Could you check a few things on this model? Use its own coordinates, in mm. Face numbers are marked on the shaded views. A direction names the side the tool comes from. Round coordinates to 2 decimals unless told otherwise and drop trailing zeros. Write each loop counter-clockwise with the first axis right and the second up, starting at its lowest first coordinate (ties: lowest second). Pieces come first, ordered by that corner, then holes. Notation, with made-up numbers: (-26, -8) -> (-7, -8) arc R18 ccw to (-7, 6) -> close; hole circle Ø8 at (52, 42.25). An arc over 180 degrees is marked (long way). One line per question, with ' | ' between items. Start each with the question number.
1. For pin 1 Ø2 at (x, z) = (-171.5, 5.5) entering from -Y; pin 2 Ø1 at (x, z) = (-159, 5.5) entering from -Y; pin 3 Ø6.5 at (y, z) = (-82.5, 6) entering from +X, each with a flat end and sliding along its axis, tell me the tip position at first contact or that it passes through.
2. If I drill on line 1 along Z through (x, y) = (-163, 104); line 2 along Y through (x, z) = (-170, 9); line 3 along X through (y, z) = (64.25, 8), over which ranges is the centre line in solid material (lowest first)? Write a range as [from, to].
3. Imagine slicing it at C-C, the plane y = -64. List the corners of the cut face in (x, z) for me.
4. For the marked faces 5, 6, 7 and 8, which set-ups out of +Z, -Z, +X, -X, +Y, -Y let a thin tool reach every point of the face, with its end or its side?
5. Imagine slicing it at B-B, the plane y = 92.5. List the corners of the cut face in (x, z) for me.
6. Thinking about a two-plate mould opening in Y: for the marked faces 1, 2, 3 and 4, which applies, released by +Y, released by -Y, zero draft, split by the parting line, or undercut?
7. Imagine slicing it at A-A, the plane y = 59.5. List the corners of the cut face in (x, z) for me.
from build123d import *

# Parameters (mm, degrees)
F0_R     = 2.1
F1_DEPTH = 16
F2_SIZE  = 2
F4_DEPTH = 3.1
F6_DEPTH = 12
F7_R     = 2
F8_DEPTH = 256.101


with BuildPart() as f1:
    # F0 (on Top) → F1 (new body)
    with BuildSketch(Plane.XY):
        with BuildLine():
            Line((-171.5, 129), (-174.5, 129))
            ThreePointArc((-174.5, 129), (-182.985281, 125.485281), (-186.5, 117))
            Line((-186.5, 117), (-186.5, -117))
            ThreePointArc((-186.5, -117), (-182.985281, -125.485281), (-174.5, -129))
            Line((-174.5, -129), (-171.5, -129))
            Line((-171.5, -129), (-171.5, -127.73274))
            Line((-171.5, -127.73274), (-171.5, -116))
            ThreePointArc((-171.5, -116), (-170.914214, -114.585786), (-169.5, -114))
            Line((-169.5, -114), (-168.828427, -114))
            ThreePointArc((-168.828427, -114), (-168.06306, -113.847759), (-167.414214, -113.414214))
            Line((-167.414214, -113.414214), (-164.414214, -110.414214))
            ThreePointArc((-164.414214, -110.414214), (-163, -109.828427), (-161.585786, -110.414214))
            Line((-161.585786, -110.414214), (-158.585786, -113.414214))
            ThreePointArc((-158.585786, -113.414214), (-157.93694, -113.847759), (-157.171573, -114))
            Line((-157.171573, -114), (-154.5, -114))
            Line((-154.5, -114), (-154.5, -99))
            Line((-154.5, -99), (-171.5, -99))
            Line((-171.5, -99), (-171.5, -72))
            Line((-171.5, -72), (-154.5, -72))
            Line((-154.5, -72), (-154.5, -56))
            Line((-154.5, -56), (-171.5, -56))
            Line((-171.5, -56), (-171.5, 56))
            Line((-171.5, 56), (-154.5, 56))
            Line((-154.5, 56), (-154.5, 72))
            Line((-154.5, 72), (-171.5, 72))
            Line((-171.5, 72), (-171.5, 99))
            Line((-171.5, 99), (-154.5, 99))
            Line((-154.5, 99), (-154.5, 114))
            Line((-154.5, 114), (-157.171573, 114))
            ThreePointArc((-157.171573, 114), (-157.93694, 113.847759), (-158.585786, 113.414214))
            Line((-158.585786, 113.414214), (-161.585786, 110.414214))
            ThreePointArc((-161.585786, 110.414214), (-163, 109.828427), (-164.414214, 110.414214))
            Line((-164.414214, 110.414214), (-167.414214, 113.414214))
            ThreePointArc((-167.414214, 113.414214), (-168.06306, 113.847759), (-168.828427, 114))
            Line((-168.828427, 114), (-169.5, 114))
            ThreePointArc((-169.5, 114), (-170.914214, 114.585786), (-171.5, 116))
            Line((-171.5, 116), (-171.5, 127.73274))
            Line((-171.5, 127.73274), (-171.5, 129))
        make_face()
        with Locations((-166.5, -64)):
            Circle(F0_R, mode=Mode.SUBTRACT)
        with Locations((-166.5, 64)):
            Circle(F0_R, mode=Mode.SUBTRACT)
    extrude(amount=F1_DEPTH)

    # F2
    f2_edges = [f1.edges().sort_by_distance(p)[0] for p in [
        (-173, -129, 16),
    ]]
    chamfer(f2_edges, length=F2_SIZE)

    # F3 (on face) → F4 (cut)
    with BuildSketch(Plane.XY.offset(16)):
        with BuildLine():
            ThreePointArc((-174.5, 125), (-180.156854, 122.656854), (-182.5, 117))
            Line((-182.5, 117), (-182.5, -117))
            ThreePointArc((-182.5, -117), (-180.156854, -122.656854), (-174.5, -125))
            Line((-174.5, -125), (-154.5, -125))
            Line((-154.5, -125), (-153.811902, 125))
            Line((-153.811902, 125), (-174.5, 125))
        make_face()
    extrude(amount=-F4_DEPTH, mode=Mode.SUBTRACT)

    # F5 (on face) → F6 (cut)
    with BuildSketch(Plane.XY):
        with BuildLine():
            ThreePointArc((-184.6, 115.1), (-181.085281, 123.585281), (-172.6, 127.1))
            Line((-172.6, 127.1), (-152.206928, 127.1))
            Line((-152.206928, 127.1), (-152.206928, 132.1))
            Line((-152.206928, 132.1), (-172.6, 132.1))
            ThreePointArc((-172.6, 132.1), (-184.620815, 127.120815), (-189.6, 115.1))
            Line((-189.6, 115.1), (-189.6, -115.1))
            ThreePointArc((-189.6, -115.1), (-184.620815, -127.120815), (-172.6, -132.1))
            Line((-172.6, -132.1), (-152.206928, -132.1))
            Line((-152.206928, -132.1), (-152.206928, -127.1))
            Line((-152.206928, -127.1), (-172.6, -127.1))
            ThreePointArc((-172.6, -127.1), (-181.085281, -123.585281), (-184.6, -115.1))
            Line((-184.6, -115.1), (-184.6, 115.1))
        make_face()
    extrude(amount=F6_DEPTH, mode=Mode.SUBTRACT)

    # F7 (on face) → F8 (cut, through all)
    with BuildSketch(Plane.XZ.offset(127.1)):
        with Locations((-163, 8)):
            Circle(F7_R)
        with Locations((163, 8)):
            Circle(F7_R)
    extrude(amount=-F8_DEPTH, mode=Mode.SUBTRACT)


solid = f1.part
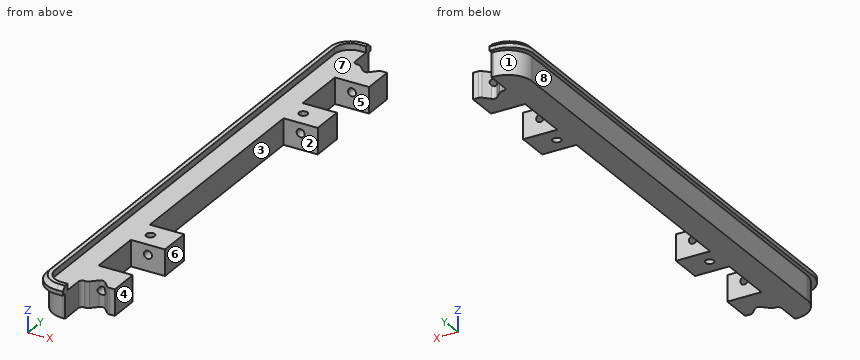
Geometry results:
1) pin 1: stops at y = -127.1 | pin 2: stops at y = -113.5 | pin 3: stops at x = -171.5
2) line 1: z = [0, 6], [10, 12.9] | line 2: y = [-114.06, -99], [-72, -56], [56, 72], [99, 114.06] | line 3: x = [-184.6, -168.59], [-161, -154.5]
3) outline: (-186.5, 12) -> (-184.6, 12) -> (-184.6, 0) -> (-168.6, 0) -> (-168.6, 12.9) -> (-182.5, 12.9) -> (-182.5, 16) -> (-184.5, 16) -> (-186.5, 14) -> close; (-164.4, 0) -> (-154.5, 0) -> (-154.5, 12.9) -> (-164.4, 12.9) -> (-164.4, 9.43) arc R2 cw (long way) to (-164.4, 6.57) -> close
4) face 5: +Z, -Z, +X | face 6: +Z, -Z, +X, +Y, -Y | face 7: +Z, +X | face 8: -Z, -X, +Y, -Y
5) outline: (-186.5, 12) -> (-184.6, 12) -> (-184.6, 0) -> (-171.5, 0) -> (-171.5, 12.9) -> (-182.5, 12.9) -> (-182.5, 16) -> (-184.5, 16) -> (-186.5, 14) -> close
6) face 1: released by +Y | face 2: undercut | face 3: undercut | face 4: zero draft
7) outline: (-186.5, 12) -> (-184.6, 12) -> (-184.6, 0) -> (-154.5, 0) -> (-154.5, 12.9) -> (-182.5, 12.9) -> (-182.5, 16) -> (-184.5, 16) -> (-186.5, 14) -> close; hole circle Ø4 at (-163, 8)
